CAD build for the part. Positions are in the model's coordinates, mm. A direction names the side the tool comes from. Round coordinates to 2 decimals unless told otherwise and drop trailing zeros. Loops run counter-clockwise (first coordinate to the right, second up) from the corner with the lowest first, then second, coordinate; pieces in that order, holes last. Notation, with made-up numbers: M 85,44 L 109,44 A15 cw 109,61 Z; hole C 83.25,41 d8. An arc over 180 degrees is marked long. One line per item, written item: value. Start each with the question number.
from build123d import *

# Parameters (mm, degrees)
SKETCH_1_R           = 4.5
EXTRUDE_4_DEPTH      = 5
SKETCH_3_R           = 5.35
CUT_EXTRUDE_3_DEPTH  = 4
SKETCH_11_R          = 1.5
CUT_EXTRUDE_13_DEPTH = 214.834047803
SKETCH_12_W          = 20
SKETCH_12_H          = 5
CUT_EXTRUDE_14_DEPTH = 2
SKETCH_13_W          = 20
SKETCH_13_H          = 5
CUT_EXTRUDE_15_DEPTH = 2
SKETCH_14_R          = 2.1
CUT_EXTRUDE_17_DEPTH = 214.834047803
SKETCH_15_W          = 20.5
SKETCH_15_H          = 40.5
CUT_EXTRUDE_18_DEPTH = 2


with BuildPart() as part:
    # 草图1 → 凸台-拉伸4 (new body)
    with BuildSketch(Plane.XY):
        with BuildLine():
            ThreePointArc((-6.801514389, 18.807961134), (-20, 0), (-6.801514389, -18.807961134))
            Line((-6.801514389, -18.807961134), (51.8, -40))
            Line((51.8, -40), (138.2, -40))
            Line((138.2, -40), (196.801514389, -18.807961134))
            ThreePointArc((196.801514389, -18.807961134), (210, 0), (196.801514389, 18.807961134))
            Line((196.801514389, 18.807961134), (138.2, 40))
            Line((138.2, 40), (51.8, 40))
            Line((51.8, 40), (-6.801514389, 18.807961134))
        make_face()
        with Locations((73.4, 0)):
            Circle(SKETCH_1_R, mode=Mode.SUBTRACT)
        Circle(SKETCH_1_R, mode=Mode.SUBTRACT)
        with Locations((116.6, 0)):
            Circle(SKETCH_1_R, mode=Mode.SUBTRACT)
        with Locations((190, 0)):
            Circle(SKETCH_1_R, mode=Mode.SUBTRACT)
    extrude(amount=EXTRUDE_4_DEPTH)

    # 草图3 → 切除-拉伸3 (cut)
    with BuildSketch(Plane.XY.offset(5)):
        Circle(SKETCH_3_R)
        with Locations((190, 0)):
            Circle(SKETCH_3_R)
    extrude(amount=-CUT_EXTRUDE_3_DEPTH, mode=Mode.SUBTRACT)

    # 草图11 → 切除-拉伸13 (cut, through all)
    with BuildSketch(Plane.XY.offset(5)):
        with Locations((100, 33.790093942)):
            Circle(SKETCH_11_R)
        with Locations(Location((90, 33.790093942, 0), (0, 0, 180))):
            Circle(SKETCH_11_R)
        with Locations(Location((100, -33.790093942, 0), (0, 0, 180))):
            Circle(SKETCH_11_R)
        with Locations((90, -33.790093942)):
            Circle(SKETCH_11_R)
    extrude(amount=-CUT_EXTRUDE_13_DEPTH, mode=Mode.SUBTRACT)

    # 草图12 → 切除-拉伸14 (cut)
    with BuildSketch(Plane.XY.offset(5)):
        with Locations((95, 33.790093942)):
            Rectangle(SKETCH_12_W, SKETCH_12_H)
        with Locations((95, -33.790093942)):
            Rectangle(SKETCH_12_W, SKETCH_12_H)
    extrude(amount=-CUT_EXTRUDE_14_DEPTH, mode=Mode.SUBTRACT)

    # 草图13 → 切除-拉伸15 (cut)
    with BuildSketch(Plane(origin=(0, 0, 0), x_dir=(-1, 0, 0), z_dir=(0, 0, -1))):
        with Locations((-95, 33.790093942)):
            Rectangle(SKETCH_13_W, SKETCH_13_H)
        with Locations((-95, -33.790093942)):
            Rectangle(SKETCH_13_W, SKETCH_13_H)
    extrude(amount=-CUT_EXTRUDE_15_DEPTH, mode=Mode.SUBTRACT)

    # 草图14 → 切除-拉伸17 (cut, through all)
    with BuildSketch(Plane.XY.offset(5)):
        with Locations((78.4, -35)):
            Circle(SKETCH_14_R)
        with Locations((78.4, 15)):
            Circle(SKETCH_14_R)
        with Locations(Location((68.4, -35, 0), (0, 0, 180))):
            Circle(SKETCH_14_R)
        with Locations((111.6, -35)):
            Circle(SKETCH_14_R)
        with Locations((121.6, -35)):
            Circle(SKETCH_14_R)
        with Locations(Location((68.4, 15, 0), (0, 0, 180))):
            Circle(SKETCH_14_R)
        with Locations((111.6, 15)):
            Circle(SKETCH_14_R)
        with Locations((121.6, 15)):
            Circle(SKETCH_14_R)
    extrude(amount=-CUT_EXTRUDE_17_DEPTH, mode=Mode.SUBTRACT)

    # 草图15 → 切除-拉伸18 (cut)
    with BuildSketch(Plane.XY.offset(5)):
        with Locations((73.4, -10)):
            Rectangle(SKETCH_15_W, SKETCH_15_H)
        with Locations((116.6, -10)):
            Rectangle(SKETCH_15_W, SKETCH_15_H)
    extrude(amount=-CUT_EXTRUDE_18_DEPTH, mode=Mode.SUBTRACT)


solid = part.part
(1) Slice it at A-A, the plane x = 116.6. List the corners of the cut face in (y, z), and give its area (3 significant figures).
(2) Probe L1, parallel to Y at x = 100, z = 2.85; L2, parallel to X at y = -13, z = 3.85; L3, parallel to X at y = 1.5, z = 2.5. List the from-to ranges inside material, lowest first.
(3) Mould opens along Y. For faces 1 (the flat face through (-3, 4, 1)), 2 (the flat face through (93, 1, 0)), 3 (the flat face through (167.091, -29.552, 2.465)), 4 (the flat face through (96, 40, 2)) say: pulls with the +Y half, pulls with the -Y half, needs draft (parallel to the pull), parting line crosses it, or undercut.
(4) Slice it at C-C, the plane x = 190. List the corners of the cut face in (y, z).
(5) Slice it at B-B, the plane y = 15. List the corners of the cut face in (x, z).
(6) Which spindle directions (+Z, -Z, +X, -X, +Y, -Y) get a long thin tool onto all of the face, cutting with end or side? Do faces 5 (the flat face through (93, 1, 5)), 6 (the flat face through (95, 34, 2)), 7 (the flat face through (116, -10, 3)). Say none if no direction does.
(7) Flat gauge pins, fed straight in: P1, Ø3, axis at y = -3.5, z = 2.5, coming from the +X side; P2, Ø3.5, axis at x = 90, y = 33.79, coming from the -Z side; P3, Ø16.5, axis at x = 73, y = -11, coming from the +Z side. Where does each tip first touch, or does it go through?
(8) Slice it at D-D, the plane y = 0. Count the separate pieces of the cut face and the enclosed holes in it, and give its area (3 significant figures).
Check result:
1. outline: M -40,0 L -4.5,0 L -4.5,3 L -30.25,3 L -30.25,5 L -40,5 Z; M 4.5,0 L 40,0 L 40,5 L 10.25,5 L 10.25,3 L 4.5,3 Z
1. area: 292 mm^2
2. L1: y = -40 to -35.29, -32.29 to 32.29, 35.29 to 40
2. L2: x = -15.2 to 63.15, 83.65 to 106.35, 126.85 to 205.2
2. L3: x = -19.94 to -5.14, 5.14 to 69.16, 77.64 to 112.36, 120.84 to 184.86, 195.14 to 209.94
3. face 1: undercut
3. face 2: needs draft
3. face 3: pulls with the -Y half
3. face 4: pulls with the +Y half
4. outline: M -21.27,0 L -4.5,0 L -4.5,1 L -5.35,1 L -5.35,5 L -21.27,5 Z; M 4.5,0 L 21.27,0 L 21.27,5 L 5.35,5 L 5.35,1 L 4.5,1 Z
5. outline: M -13.23,0 L 66.3,0 L 66.3,5 L -13.23,5 Z; M 70.5,0 L 76.3,0 L 76.3,5 L 70.5,5 Z; M 80.5,0 L 109.5,0 L 109.5,5 L 80.5,5 Z; M 113.7,0 L 119.5,0 L 119.5,5 L 113.7,5 Z; M 123.7,0 L 203.23,0 L 203.23,5 L 123.7,5 Z
6. face 5: +Z, +X, -X, +Y, -Y
6. face 6: -Z
6. face 7: +Z
7. P1: stops at x = 209.9
7. P2: stops at z = 2
7. P3: stops at z = 3
8. separate pieces: 5
8. enclosed holes: 0
8. area: 910 mm^2
